Check sheet for the modelled part. Datum: model origin and axes. Units: mm. Coordinates: 2 decimals unless noted, no trailing zeros. Order: outer loops, then holes, each group sorted by start corner. A loop starts at its lowest first (then second) coordinate and runs counter-clockwise, first axis right, second up.
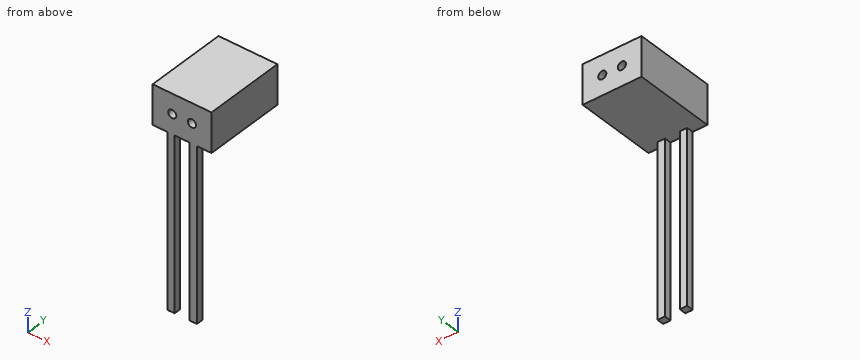
from build123d import *

# Parameters (mm, degrees)
SKETCH2_W             = 3
SKETCH2_H             = 2.8
BOSS_EXTRUDE1_DEPTH   = 70
BOSS_EXTRUDE1_2_DEPTH = 70
SKETCH3_W             = 24
SKETCH3_H             = 33.2
BOSS_EXTRUDE2_DEPTH   = 16
SKETCH4_R             = 1.65
CUT_EXTRUDE1_DEPTH    = 34.2
CUT_EXTRUDE2_START    = 3
CUT_EXTRUDE2_DEPTH    = 2.8


with BuildPart() as part:
    # Sketch2 → Boss-Extrude1 (new body)
    with BuildSketch(Plane.XY):
        with Locations((7.466666667, 1.4)):
            Rectangle(SKETCH2_W, SKETCH2_H)
    extrude(amount=-BOSS_EXTRUDE1_DEPTH)



with BuildPart() as body_2:
    # Sketch2 → Boss-Extrude1 2 (new body)
    with BuildSketch(Plane.XY):
        with Locations((16.533333333, 1.4)):
            Rectangle(SKETCH2_W, SKETCH2_H)
    extrude(amount=-BOSS_EXTRUDE1_2_DEPTH)


with BuildPart() as part_1:
    add(part.part)

    add(body_2.part)  # Boss-Extrude2 merges body 2
    # Sketch3 → Boss-Extrude2 (add)
    with BuildSketch(Plane.XY):
        with Locations((12, 16.6)):
            Rectangle(SKETCH3_W, SKETCH3_H)
    extrude(amount=BOSS_EXTRUDE2_DEPTH)

    # Sketch4 → Cut-Extrude1 (cut, through all)
    with BuildSketch(Plane(origin=(0, 0, 0), x_dir=(1, 0, 0), z_dir=(0, 1, 0))):
        with Locations((8, -8)):
            Circle(SKETCH4_R)
        with Locations((16, -8)):
            Circle(SKETCH4_R)
    extrude(amount=CUT_EXTRUDE1_DEPTH, mode=Mode.SUBTRACT)

    # Sketch5 → Cut-Extrude2 (cut)
    with BuildSketch(Plane(origin=(0, 0, 0), x_dir=(1, 0, 0), z_dir=(0, 1, 0)).offset(CUT_EXTRUDE2_START)):
        Polygon((11.290896534, -8), (9.645448267, -5.15), (6.354551733, -5.15), (4.709103466, -8), (6.354551733, -10.85), (9.645448267, -10.85), align=None)
        Polygon((19.290896534, -8), (17.645448267, -5.15), (14.354551733, -5.15), (12.709103466, -8), (14.354551733, -10.85), (17.645448267, -10.85), align=None)
    extrude(amount=CUT_EXTRUDE2_DEPTH, mode=Mode.SUBTRACT)


solid = part_1.part
(1) Cross-section at A-A (z = -58). Enter the section's corners in (x, y).
Filled in:
outline: (5.97, 0) - (8.97, 0) - (8.97, 2.8) - (5.97, 2.8) - close; (15.03, 0) - (18.03, 0) - (18.03, 2.8) - (15.03, 2.8) - close
(2) Cross-section at C-C (y = 15). Enter the section's corners in (x, z), and give its area (3 significant figures).
Filled in:
outline: (0, 0) - (24, 0) - (24, 16) - (0, 16) - close; hole circle Ø3.3 at (8, 8); hole circle Ø3.3 at (16, 8)
area: 367 mm2
(3) Cross-section at D-D (x = 3.25). Enter the section's corners in (y, z).
Filled in:
outline: (0, 0) - (33.2, 0) - (33.2, 16) - (0, 16) - close
(4) Cross-section at B-B (x = 16). Enter the section's corners in (y, z), and give its area (3 significant figures).
Filled in:
outline: (0, -70) - (2.8, -70) - (2.8, 0) - (33.2, 0) - (33.2, 6.35) - (5.8, 6.35) - (5.8, 5.15) - (3, 5.15) - (3, 6.35) - (0, 6.35) - close; (0, 9.65) - (3, 9.65) - (3, 10.85) - (5.8, 10.85) - (5.8, 9.65) - (33.2, 9.65) - (33.2, 16) - (0, 16) - close
area: 611 mm2
(5) Go/stop test with flat-tipped pins: P1, Ø1, axis at x = 10, y = 12.5, coming from the -Z side; P2, Ø1.5, axis at x = 8, z = -30, coming from the +Y side; P3, Ø3, axis at x = 16, z = 8, coming from the +Y side; P4, Ø0.8, axis at y = 2, z = -42, coming from the +X side. Record where each tip stops, or that it passes through.
Filled in:
P1: stops at z = 0
P2: stops at y = 2.8
P3: passes through
P4: stops at x = 18.03
(6) Thickness scan on probe 1 along Z at (x, y) = (16, 0.7); probe 2 along Z at (x, y) = (8, 25.25); probe 3 along Y at (x, z) = (17.5, -17). Record the ranges inside material, lowest first.
Filled in:
probe 1: z = -70 to 6.35, 9.65 to 16
probe 2: z = 0 to 6.35, 9.65 to 16
probe 3: y = 0 to 2.8
